The listing builds one solid part. Answer for the finished solid, in the listing's coordinates (mm). A direction names the side the tool comes from. Round coordinates to 2 decimals unless told otherwise and drop trailing zeros. Order: outer loops, then holes, each group sorted by start corner. A loop starts at its lowest first (then second) coordinate and runs counter-clockwise, first axis right, second up. Notation, with made-up numbers: (17, 75) - (56, 75) arc R26 cw to (56, 104) - close; hole circle Ø1 at (37.5, 70.5). An arc over 180 degrees is marked (long way). Use CSV: the item, a comma, the result in double quotes. Start each with the question number.
Item 1: Find section B-B, the plane z = 5.5. Give the vertices of the cut face in (x, y), plus the area to 3 significant figures.
Item 2: For faces 4 (the flat face through (5.194, -0.751, -10.02)), 5 (the flat face through (-10, -1, 7.044)), 6 (the flat face through (9, -1, 7.044)), 7 (the flat face through (10.09, -0.75, 3.47)), determine the directions among +Z, -Z, +X, -X, +Y, -Y from which every point of the face is accessible in a straight line to the end or side of a thin tool.
Item 3: Find section A-A, the plane y = -0.4. Give the vertices of the cut face in (x, z), plus the area to 3 significant figures.
Item 4: Determine the mould class of faces 1 (the flat face through (-7.912, -0.751, -7.018)), 2 (the flat face through (-1.702, -0.751, 12.22)), 3 (the flat face through (-1, 0, 0)) for opening direction Z: +Z half, -Z half, draft (parallel to the pull), parting line (faces both ways), or undercut.
Item 5: Find section C-C, the plane x = 11.5. Give the vertices of the cut face in (y, z).
Item 6: Straight lines are drawn through the part: line 1 along X through (y, z) = (-1.15, -10); line 2 along Z through (x, y) = (-13.5, -0.2); line 3 along X through (y, z) = (-1.25, 4.5). For each, find the intervals that lie inside material, in ascending order. Write a range as [from, to].
Item 7: A flat-ended cylindrical pin translates along its axis: P1, Ø0.8, axis at x = 9, y = -1, coming from the +Z side. Find the tip coordinate at first contact, or state that the pin passes through.
```python
from build123d import *

# Parameters (mm, degrees)
F2_DEPTH = 1.524


with BuildPart() as f2:
    # F1 (on face) → F2 (new body)
    with BuildSketch(Plane.XZ):
        Polygon((3.452803, 7.043747), (0, 17.254066), (-3.452803, 7.043747), (-15.913724, 7.043747), (-5.658479, -0.034705), (-10.230287, -14.200249), (0, -5.954943), (10.535668, -14.200249), (6.072822, 0), (14.231136, 7.043747), align=None)
    extrude(amount=F2_DEPTH)


solid = f2.part
```
Worked out:
1,outline,"(-13.68, -1.52) - (12.44, -1.52) - (12.44, 0) - (-13.68, 0) - close"
1,area,"39.8 mm²"
2,face 4,"-Z, +Y, -Y"
2,face 5,"+Z, -X, +Y, -Y"
2,face 6,"+Z, +X, +Y, -Y"
2,face 7,"+X, +Y, -Y"
3,outline,"(-15.91, 7.04) - (-5.66, -0.03) - (-10.23, -14.2) - (0, -5.95) - (10.54, -14.2) - (6.07, 0) - (14.23, 7.04) - (3.45, 7.04) - (0, 17.25) - (-3.45, 7.04) - close"
3,area,"328 mm²"
4,face 1,"undercut"
4,face 2,"+Z half"
4,face 3,"draft"
5,outline,"(-1.52, 4.69) - (0, 4.69) - (0, 7.04) - (-1.52, 7.04) - close"
6,line 1,"x = [-8.87, -5.02], [5.17, 9.22]"
6,line 2,"z = [5.38, 7.04]"
6,line 3,"x = [-12.23, 11.28]"
7,P1,"stops at z = 7.04"
